Input: part model. Units: mm. Frame: model coordinates. Face numbers are marked on the shaded views. A direction names the side the tool comes from. Round coordinates to 2 decimals unless told otherwise and drop trailing zeros. Write each loop counter-clockwise with the first axis right and the second up, starting at its lowest first coordinate (ties: lowest second). Pieces come first, ordered by that corner, then holes. Notation, with made-up numbers: (39.5, 81.25) -> (81.5, 81.25) arc R21 ccw to (81.5, 101.25) -> close; hole circle Ø9 at (86, -18). An arc over 180 degrees is marked (long way). Use CSV: the item, a comma, the result in double quotes.
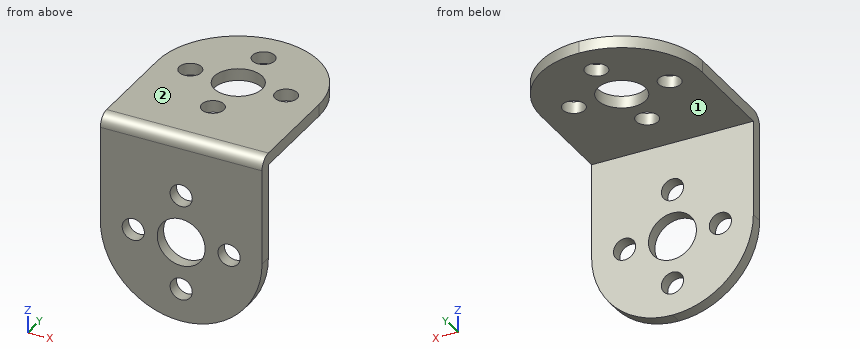
```python
from build123d import *

# Parameters (mm, degrees)
EXTRUDE1_DEPTH           = 27
CUT_EXTRUDE1_START       = -2
CUT_EXTRUDE1_OUTLINE_R   = 4
CUT_EXTRUDE1_OUTLINE_R_2 = 1.85
CUT_EXTRUDE1_DEPTH       = 2
CUT_EXTRUDE2_START       = -2
CUT_EXTRUDE2_OUTLINE_R   = 4
CUT_EXTRUDE2_OUTLINE_R_2 = 1.85
CUT_EXTRUDE2_DEPTH       = 2
FILLET1_R                = 13.5
FILLET2_R                = 13.5
FILLET3_R                = 13.5
FILLET4_R                = 13.5
FILLET5_R                = 2


# Read off the part's stored shape, not the designer's step: Cut-Extrude1, Cut-Extrude2
with BuildPart() as part:
    # Sketch1 → Extrude1 (new body)
    with BuildSketch(Plane(origin=(0, 0, 0), x_dir=(0, 0, -1), z_dir=(1, 0, 0))):
        Polygon((0, 0), (31.5, 0), (31.5, 2), (2, 2), (2, 31.5), (0, 31.5), align=None)
    extrude(amount=-EXTRUDE1_DEPTH)

    # Cut-Extrude1 outline → Cut-Extrude1 (cut)
    with BuildSketch(Plane.XY.offset(CUT_EXTRUDE1_START)):
        with Locations((-13.5, 18)):
            Circle(CUT_EXTRUDE1_OUTLINE_R)
        with Locations((-5.5, 18)):
            Circle(CUT_EXTRUDE1_OUTLINE_R_2)
        with Locations((-21.5, 18)):
            Circle(CUT_EXTRUDE1_OUTLINE_R_2)
        with Locations((-13.5, 10)):
            Circle(CUT_EXTRUDE1_OUTLINE_R_2)
        with Locations((-13.5, 26)):
            Circle(CUT_EXTRUDE1_OUTLINE_R_2)
    extrude(amount=CUT_EXTRUDE1_DEPTH, mode=Mode.SUBTRACT)

    # Cut-Extrude2 outline → Cut-Extrude2 (cut)
    with BuildSketch(Plane.XZ.offset(CUT_EXTRUDE2_START)):
        with Locations((-13.5, -18)):
            Circle(CUT_EXTRUDE2_OUTLINE_R)
        with Locations((-5.5, -18)):
            Circle(CUT_EXTRUDE2_OUTLINE_R_2)
        with Locations((-21.5, -18)):
            Circle(CUT_EXTRUDE2_OUTLINE_R_2)
        with Locations((-13.5, -26)):
            Circle(CUT_EXTRUDE2_OUTLINE_R_2)
        with Locations((-13.5, -10)):
            Circle(CUT_EXTRUDE2_OUTLINE_R_2)
    extrude(amount=CUT_EXTRUDE2_DEPTH, mode=Mode.SUBTRACT)

    # Fillet1
    fillet1_edges = [part.edges().sort_by_distance(p)[0] for p in [
        (0, 31.5, -1),
    ]]
    fillet(fillet1_edges, radius=FILLET1_R)

    # Fillet2
    fillet2_edges = [part.edges().sort_by_distance(p)[0] for p in [
        (-27, 31.5, -1),
    ]]
    fillet(fillet2_edges, radius=FILLET2_R - 0.0001)  # a hair under: the kernel refuses the full size

    # Fillet3
    fillet3_edges = [part.edges().sort_by_distance(p)[0] for p in [
        (0, 1, -31.5),
    ]]
    fillet(fillet3_edges, radius=FILLET3_R)

    # Fillet4
    fillet4_edges = [part.edges().sort_by_distance(p)[0] for p in [
        (-27, 1, -31.5),
    ]]
    fillet(fillet4_edges, radius=FILLET4_R - 0.0001)  # a hair under: the kernel refuses the full size

    # Fillet5
    fillet5_edges = [part.edges().sort_by_distance(p)[0] for p in [
        (-13.5, 0, 0),
    ]]
    fillet(fillet5_edges, radius=FILLET5_R)


solid = part.part
```
Item 1: Section query D-D on x = -14.5. Give the number of separate pieces and of enclosed holes in the cut face, plus the area to 3 significant figures.
Worked answers:
separate pieces,"7"
enclosed holes,"0"
area,"65.1 mm²"
Item 2: Section query A-A on y = 17.5. Return the cut outline in (x, z), plus the area to 3 significant figures.
Worked answers:
outline,"(-27, -2) -> (-23.28, -2) -> (-23.28, 0) -> (-27, 0) -> close; (-19.72, -2) -> (-17.47, -2) -> (-17.47, 0) -> (-19.72, 0) -> close; (-9.53, -2) -> (-7.28, -2) -> (-7.28, 0) -> (-9.53, 0) -> close; (-3.72, -2) -> (0, -2) -> (0, 0) -> (-3.72, 0) -> close"
area,"23.9 mm²"
Item 3: First-contact query: pin 1 Ø13 at (x, y) = (-13.5, 18) entering from -Z; pin 2 Ø3.5 at (x, y) = (-21.5, 18) entering from -Z; pin 3 Ø3 at (x, z) = (-24.5, -22) entering from -Y; pin 4 Ø6 at (x, z) = (-13.5, -26) entering from +Y. Flat tips, straight axial feed; report the tip coordinate or a pass-through.
Worked answers:
pin 1,"stops at z = -2"
pin 2,"passes through"
pin 3,"stops at y = 0"
pin 4,"stops at y = 2"
Item 4: Section query C-C on x = -10.5. Return the cut outline in (y, z), plus the area to 3 significant figures.
Worked answers:
outline,"(0, -31.16) -> (2, -31.16) -> (2, -20.65) -> (0, -20.65) -> close; (0, -15.35) -> (2, -15.35) -> (2, -2) -> (15.35, -2) -> (15.35, 0) -> (2, 0) arc R2 ccw to (0, -2) -> close; (20.65, -2) -> (31.16, -2) -> (31.16, 0) -> (20.65, 0) -> close"
area,"98.6 mm²"
Item 5: Set-up query: the marked faces 1 and 2. Return all of +Z, -Z, +X, -X, +Y, -Y with unobstructed straight access to the full face (end or side cutting, diameter ignored); none if empty.
Worked answers:
face 1,"-Z, +X, -X, +Y"
face 2,"+Z, +X, -X, +Y, -Y"
Item 6: Section query B-B on z = -25. Return the cut outline in (x, y).
Worked answers:
outline,"(-25.04, 0) -> (-15.06, 0) -> (-15.06, 2) -> (-25.04, 2) -> close; (-11.94, 0) -> (-1.96, 0) -> (-1.96, 2) -> (-11.94, 2) -> close"
Item 7: Line query: line 1 (Y direction, x = -25.25, z = -20); line 2 (Z direction, x = -12.25, y = 14); line 3 (Z direction, x = -5.5, y = 0.65). Output: solid intervals per line, ascending.
Worked answers:
line 1,"y = 0 to 2"
line 2,"z = -2 to 0"
line 3,"z = -28.87 to -19.85, -16.15 to -0.52"
